Part model, mm, in its own coordinate system. Coordinates: 2 decimals unless noted, no trailing zeros. Loops run counter-clockwise (first coordinate to the right, second up) from the corner with the lowest first, then second, coordinate; pieces in that order, holes last. Notation, with made-up numbers: (-40, -22) - (0, -22) arc R23 cw to (0, 1) - close; hole circle Ø10 at (-16, -8.75). An arc over 180 degrees is marked (long way). Use a Markdown table: item, result. Add a question column.
1. Band-saw the part on A-A, the plane z = 0.7. Give the cut face in (x, y).
2. Band-saw the part on C-C, the plane y = -90. Give the cut face in (x, z).
3. Band-saw the part on D-D, the plane y = -65.5. Give the cut face in (x, z).
4. Wall check: probe 1 along X at (y, z) = (-29, 1.4); probe 2 along X at (y, z) = (-14.5, 0.9); probe 3 along Y at (x, z) = (18, 0.2). Give the ranges that are in metal, low to high. Write a range as [from, to].
5. Band-saw the part on B-B, the plane x = 17. Give the cut face in (y, z), plus the area to 3 significant figures.
6. Drop a flat-ended pin along its axis: pin 1 (1 mm diameter, centred on y = -5, z = 1.5, fed in from -X). Give the stop position or say it passes through.
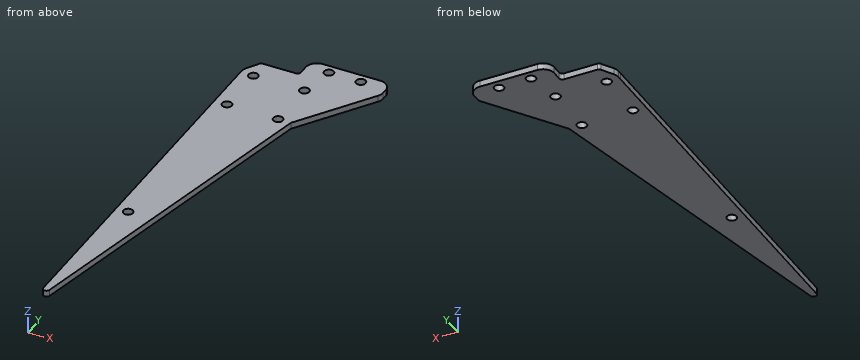
from build123d import *

# Parameters (mm, degrees)
EXTRUDE_1_DEPTH     = 2
SKETCH_2_R          = 1.5
CUT_EXTRUDE_1_DEPTH = 5
SKETCH_3_R          = 1.5
CUT_EXTRUDE_2_DEPTH = 10
FILLET_1_R          = 3.5
FILLET_2_R          = 1
SKETCH_4_R          = 1.5
EXTRUDE_2_DEPTH     = 2


with BuildPart() as part:
    # 草图1 → 凸台-拉伸1 (new body)
    with BuildSketch(Plane.XY):
        Polygon((5, -36), (-15, -16), (-15, -12.5), (-12, -7.5), (0, -7.5), (0, 0), (25, 0), (25, -6), align=None)
    extrude(amount=EXTRUDE_1_DEPTH)

    # 草图2 → 切除-拉伸1 (cut)
    with BuildSketch(Plane.XY.offset(2)):
        with Locations((17, -3)):
            Circle(SKETCH_2_R)
        with Locations((7, -3)):
            Circle(SKETCH_2_R)
    extrude(amount=-CUT_EXTRUDE_1_DEPTH, mode=Mode.SUBTRACT)

    # 草图3 → 切除-拉伸2 (cut)
    with BuildSketch(Plane.XY.offset(2)):
        with Locations((5, -30)):
            Circle(SKETCH_3_R)
        with Locations((5, -14)):
            Circle(SKETCH_3_R)
        with Locations((-11, -14)):
            Circle(SKETCH_3_R)
    extrude(amount=-CUT_EXTRUDE_2_DEPTH, mode=Mode.SUBTRACT)

    # 圆角1
    fillet_1_edges = [part.edges().sort_by_distance(p)[0] for p in [
        (25, 0, 1),
        (25, -6, 1),
        (5, -36, 1),
        (-15, -16, 1),
        (-15, -12.5, 1),
        (0, 0, 1),
    ]]
    fillet(fillet_1_edges, radius=FILLET_1_R)

    # 圆角2
    fillet_2_edges = [part.edges().sort_by_distance(p)[0] for p in [
        (-12, -7.5, 1),
        (0, -7.5, 1),
    ]]
    fillet(fillet_2_edges, radius=FILLET_2_R)

    # 草图4 → 凸台-拉伸2 (add)
    with BuildSketch(Plane.XY.offset(2)):
        with BuildLine():
            Line((9, -30), (-12.660289895, -134.591804029))
            ThreePointArc((-12.660289895, -134.591804029), (-13.739948562, -135.383956892), (-14.639507537, -134.392007979))
            Line((-14.639507537, -134.392007979), (-15, -14.009848205))
            Line((-15, -14.009848205), (9, -30))
        make_face()
        with Locations((-11, -30)):
            Circle(SKETCH_4_R, mode=Mode.SUBTRACT)
        with Locations((-11, -90)):
            Circle(SKETCH_4_R, mode=Mode.SUBTRACT)
        with Locations((5, -30)):
            Circle(SKETCH_4_R, mode=Mode.SUBTRACT)
    extrude(amount=-EXTRUDE_2_DEPTH)


solid = part.part
Geometry check:
| question | item | result |
|---|---|---|
| 1 | outline | (-15, -14.67) - (-14.64, -134.39) arc R1 ccw to (-12.66, -134.59) - (9, -30) - (24.41, -6.88) arc R3.5 ccw to (25, -4.94) - (25, -3.5) arc R3.5 ccw to (21.5, 0) - (3.5, 0) arc R3.5 ccw to (0, -3.5) - (0, -6.5) arc R1 cw to (-1, -7.5) - (-11.43, -7.5) arc R1 ccw to (-12.29, -7.99) - (-14.5, -11.67) arc R3.5 ccw to (-15, -13.47) - (-15, -14.55) arc R3.5 ccw to start; hole circle Ø3 at (-11, -90); hole circle Ø3 at (-11, -30); hole circle Ø3 at (-11, -14); hole circle Ø3 at (5, -30); hole circle Ø3 at (5, -14); hole circle Ø3 at (7, -3); hole circle Ø3 at (17, -3) |
| 2 | outline | (-14.77, 0) - (-12.5, 0) - (-12.5, 2) - (-14.77, 2) - close; (-9.5, 0) - (-3.43, 0) - (-3.43, 2) - (-9.5, 2) - close |
| 3 | outline | (-14.85, 0) - (1.65, 0) - (1.65, 2) - (-14.85, 2) - close |
| 4 | probe 1 | x = [-14.96, -12.12], [-9.88, 3.88], [6.12, 9.67] |
| 4 | probe 2 | x = [-15, -12.41], [-9.59, 3.59], [6.41, 19.33] |
| 4 | probe 3 | y = [-16.5, -4.12], [-1.88, 0] |
| 5 | outline | (-18, 0) - (-4.5, 0) - (-4.5, 2) - (-18, 2) - close; (-1.5, 0) - (0, 0) - (0, 2) - (-1.5, 2) - close |
| 5 | area | 30.0 mm^2 |
| 6 | pin 1 | stops at x = 0 |
